Here's how the part is built. I have some questions about the finished solid (model axes, mm). A direction names the side the tool comes from. Round coordinates to 2 decimals unless told otherwise and drop trailing zeros. Order: outer loops, then holes, each group sorted by start corner. A loop starts at its lowest first (then second) coordinate and runs counter-clockwise, first axis right, second up.
```python
from build123d import *

# Parameters (mm, degrees)
BOSS_EXTRU_2_DEPTH      = 9
ENL_V_MAT_EXTRU_2_DEPTH = 9
ESQUISSE5_W             = 6
ESQUISSE5_H             = 25.84965
ENL_V_MAT_EXTRU_3_DEPTH = 10


with BuildPart() as part:
    # Esquisse2 → Boss.-Extru.2 (new body)
    with BuildSketch(Plane.XY):
        with BuildLine():
            Line((0, 0), (-1055.446290734, 0))
            add(Edge.make_bspline(
                [(-1055.446290734, 0), (-1207.572733387, 59.072106031), (-1304.579199027, 189.593529265)],
                knots=[0, 0, 0, 1, 1, 1], degree=2))
            Line((-1304.579199027, 189.593529265), (-1328.155601237, 242.090877604))
            Line((-1328.155601237, 242.090877604), (-1348.517039509, 262.446992266))
            Line((-1348.517039509, 262.446992266), (-1348.517039509, 299.331021292))
            Line((-1348.517039509, 299.331021292), (-1337.24264668, 310.608362644))
            Line((-1337.24264668, 310.608362644), (-1275.966827179, 302.644588826))
            add(Edge.make_bspline(
                [(-1275.966827179, 302.644588826), (-1212.760641583, 141.531535954), (-1050.525159664, 78.394553502)],
                knots=[0, 0, 0, 1, 1, 1], degree=2))
            Line((-1050.525159664, 78.394553502), (-46.371074076, 78.394553502))
            Line((-46.371074076, 78.394553502), (48.76008987, 228.44376205))
            Line((48.76008987, 228.44376205), (115.880348206, 284.547364773))
            Line((115.880348206, 284.547364773), (175.286334456, 328.432610938))
            Line((175.286334456, 328.432610938), (175.286334456, 257.621549377))
            Line((175.286334456, 257.621549377), (107.11594567, 180.577636332))
            Line((107.11594567, 180.577636332), (0, 0))
        make_face()
    extrude(amount=BOSS_EXTRU_2_DEPTH)

    # Esquisse4 → Enlèv. mat.-Extru.2 (cut)
    with BuildSketch(Plane.XY.offset(9)):
        Polygon((-1192.710056644, 217.724215408), (-1192.710056644, 117.812636738), (-1186.710056644, 117.812636738), (-1186.710056644, 209.090265158), (-1144.70133954, 205.492785887), (-1111.824911273, 179.590935136), (-1111.824911273, 55.314515649), (-1105.824911273, 55.314515649), (-1105.824911273, 174.913937406), (-1058.771084869, 188.659470271), (-1027.191161845, 161.497477767), (-1027.191161845, 30), (-1021.191161845, 30), (-1021.191161845, 167.225098507), (-976.159938867, 174.429619005), (-943.229008237, 161.127659365), (-943.229008237, 30), (-937.229008237, 30), (-937.229008237, 164.093815562), (-899.191490776, 172.001101596), (-861.857811784, 160.098627493), (-861.857811784, 30), (-855.857811784, 30), (-855.857811784, 196.236545153), (-815.986169177, 204.901610664), (-775.188433973, 184.176190605), (-775.188433973, 30), (-769.188433973, 30), (-769.188433973, 176.450577912), (-732.223715867, 183.004336583), (-693.639593808, 163.215620457), (-693.639593808, 30), (-687.639593808, 30), (-687.639593808, 172.485228345), (-653.152535866, 182.871939208), (-610.716601792, 161.453305285), (-610.716601792, 30), (-604.716601792, 30), (-604.716601792, 256.125318922), (-551.321272632, 268.910222611), (-528.666744333, 255.862211449), (-528.666744333, 34.3), (-522.666744333, 34.3), (-522.666744333, 255.102102604), (-476.392141731, 269.107524931), (-444.607914754, 258.656296952), (-444.607914754, 36.7), (-438.607914754, 36.7), (-438.607914754, 253.443093933), (-391.056155042, 266.894918017), (-360.02126631, 254.206439852), (-360.02126631, 30), (-354.02126631, 30), (-354.02126631, 250.104032237), (-303.804875297, 262.547483763), (-275.81856885, 247.243298089), (-275.81856885, 39.1), (-269.81856885, 39.1), (-269.81856885, 230.071554094), (-217.437093626, 257.378680484), (-192.806508582, 246.762372601), (-192.806508582, 38.7), (-186.806508582, 38.7), (-186.806508582, 245.622867868), (-134.999273909, 264.79720393), (-106.993498927, 255.334085011), (-106.993498927, 46.1), (-100.993498927, 46.1), (-100.993498927, 258.655280604), (-22.735685337, 264.839286488), (-22.735685337, 88.7), (-16.735685337, 88.7), (-16.735685337, 231.395876397), (-1.733463181, 266.202092714), (54.176868866, 313.052154508), (54.176868866, 197.147050424), (60.176868866, 197.147050424), (60.176868866, 330.337520125), (-1075.947973634, 334.662873451), align=None)
    extrude(amount=-ENL_V_MAT_EXTRU_2_DEPTH, mode=Mode.SUBTRACT)

    # Esquisse5 → Enlèv. mat.-Extru.3 (cut)
    with BuildSketch(Plane.XY.offset(9)):
        Polygon((169.286334456, 324.000204482), (169.286334456, 281.800204482), (175.286334456, 281.800204482), (202.680394495, 285.052171219), (208.588297758, 339.079823363), (181.275473189, 338.718158681), align=None)
        with Locations((-1285.723549311, 291.377704112)):
            Rectangle(ESQUISSE5_W, ESQUISSE5_H)
    extrude(amount=-ENL_V_MAT_EXTRU_3_DEPTH, mode=Mode.SUBTRACT)


solid = part.part
```
1. If we mould it in two halves opening along X, with no side actions, what happens to faces 3 (the flat face through (-583, 55, 9)), 4 (the flat face through (142.21, 304, 4.44)), 5 (the flat face through (-1316.2, 215.47, 4.44))? For each: released by +X, released by -X, zero draft, split by the parting line, or undercut.
Evaluation:
face 3: zero draft
face 4: undercut
face 5: released by -X
2. If we section it at B-B, the plane y = 213: State how many separate pieces and enclosed holes the cut face has, and give its area (3 significant figures).
Evaluation:
separate pieces: 3
enclosed holes: 0
area: 1,600 mm2
3. If we section it at A-A, the plane x = -888: Write out the boundary of the cut face in (y, z), and give its area (3 significant figures).
Evaluation:
outline: (0, 0) - (78.39, 0) - (78.39, 9) - (0, 9) - close
area: 706 mm2
4. I need wall thicknesses on probe 1 along X at (y, z) = (152, 5.25); probe 2 along X at (y, z) = (278.5, 4.75); probe 3 along Y at (x, z) = (-208, 3.5). Which ranges of each line are inside material? Lowest first, please.
Evaluation:
probe 1: x = -1274.2 to -1192.71, -1186.71 to -1173.09, 0.29 to 90.16
probe 2: x = -1348.52 to -1288.72, -1282.72 to -1265.69, 108.65 to 175.29
probe 3: y = 0 to 78.39
5. I'm going to push flat-ended pins straight in: P1, Ø3, axis at y = 208, z = 2.5, coming from the +X side; P2, Ø4.5, axis at y = 78.5, z = 5, coming from the +X side; P3, Ø2.5, axis at y = 145, z = 5, coming from the +X side. Where does each tip first touch, or does it pass through?
Evaluation:
P1: stops at x = 132.71
P2: stops at x = 47.9
P3: stops at x = 86.75
6. On a 3-axis mill with a long thin cutter (end or side, diameter ignored), from which of +Z, -Z, +X, -X, +Y, -Y can I reach the whole of each face in a straight line? I mean faces 1 (the flat face through (54.308, 91.553, 4.437)), 2 (the flat face through (15.554, 176.068, 4.437)). Say none if no direction works.
Evaluation:
face 1: +Z, -Z, +X, -Y
face 2: +Z, -Z, +Y
